Check sheet for the drawn part. Datum: minimum x, y, z corner. Units: mm. Coordinates: 2 decimals unless noted, no trailing zeros. Loops run counter-clockwise (first coordinate to the right, second up) from the corner with the lowest first, then second, coordinate; pieces in that order, holes last. Notation, with made-up numbers: (15, 39) - (73, 39) arc R32 ccw to (73, 78) - close; hole circle Ø1 at (42, -11). An arc over 180 degrees is marked (long way). Answer as CSV lines item,"result". Start each with the question number.
1. Material ranges on line 1 (Y direction, x = 2.8, z = 4.75); line 2 (Y direction, x = 30, z = 4), recorded low to high. Write a range as [from, to].
2. Cross-section at B-B (z = 8.5). State how many separate pieces and enclosed holes the cut face has, plus the area to 3 significant figures.
3. Gauge pin test, flat end, axial feed: P1, Ø2, axis at x = 94.6, y = 26.3, coming from the +Z side. Record the tip position at first contact, or that the pin passes through.
4. Cross-section at A-A (x = 94.6). Enter the section's corners in (y, z).
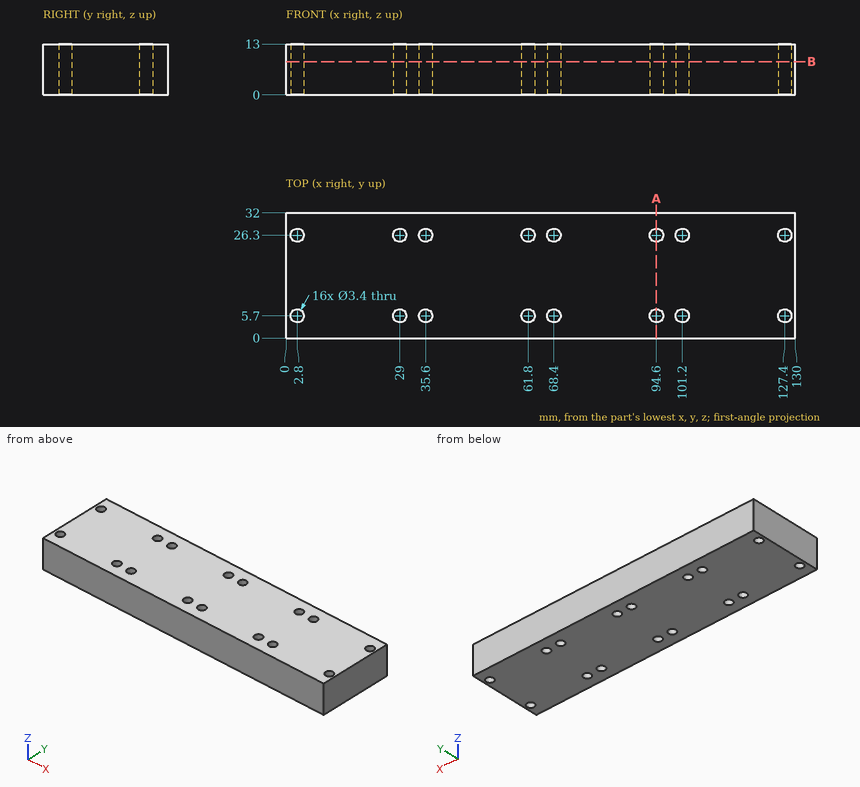
Values follow:
1,line 1,"y = [0, 4], [7.4, 24.6], [28, 32]"
1,line 2,"y = [0, 4.33], [7.07, 24.93], [27.67, 32]"
2,separate pieces,"1"
2,enclosed holes,"16"
2,area,"4,010 mm²"
3,P1,"passes through"
4,outline,"(0, 0) - (4, 0) - (4, 13) - (0, 13) - close; (7.4, 0) - (24.6, 0) - (24.6, 13) - (7.4, 13) - close; (28, 0) - (32, 0) - (32, 13) - (28, 13) - close"
